from build123d import *

# Parameters (mm, degrees)
SKETCH_1_R      = 4.025
EXTRUDE_1_DEPTH = 1.5
FILLET_1_R      = 13
FILLET_2_R      = 6
FILLET_3_R      = 1
FILLET_7_R      = 3


with BuildPart() as part:
    # 草图1 → 凸台-拉伸1 (new, symmetric)
    with BuildSketch(Plane.XY):
        with BuildLine():
            Line((38, 14.000000007), (250, 10.55184781))
            ThreePointArc((250, 10.55184781), (369.998701007, 8.688014918), (490.000004009, 7))
            ThreePointArc((490.000004009, 7), (564.99833736, 6.250002778), (640.000004009, 6))
            Line((640.000004009, 6), (750.000004009, 6))
            ThreePointArc((750.000004009, 6), (767.416160301, 6.375174017), (784.800004009, 7.5))
            ThreePointArc((784.800004009, 7.5), (788.089261415, 6.498216371), (789.772556789, 3.5))
            ThreePointArc((789.772556789, 3.5), (790.000004009, 0), (789.772556789, -3.5))
            ThreePointArc((789.772556789, -3.5), (788.089261415, -6.498216371), (784.800004009, -7.5))
            ThreePointArc((784.800004009, -7.5), (767.416160301, -6.375174017), (750.000004009, -6))
            Line((750.000004009, -6), (640.000004009, -6))
            ThreePointArc((640.000004009, -6), (564.99833736, -6.250002778), (490.000004009, -7))
            ThreePointArc((490.000004009, -7), (369.998701007, -8.688014918), (250, -10.55184781))
            Line((250, -10.55184781), (38, -14.000000007))
            Line((38, -14.000000007), (30.845299463, -26.392304848))
            Line((30.845299463, -26.392304848), (26, -18))
            Line((26, -18), (14.154700538, -38.516660498))
            Line((14.154700538, -38.516660498), (24.248711306, -56))
            Line((24.248711306, -56), (29.856406461, -56))
            Line((29.856406461, -56), (35.052558882, -65))
            Line((35.052558882, -65), (19.052558883, -65))
            Line((19.052558883, -65), (3.649147039, -38.320508076))
            Line((3.649147039, -38.320508076), (-0.207259422, -45))
            Line((-0.207259422, -45), (2.596588156, -49.856406461))
            Line((2.596588156, -49.856406461), (-2.599564267, -58.856406461))
            Line((-2.599564267, -58.856406461), (-10.599564267, -45))
            Line((-10.599564267, -45), (-1.547005384, -29.320508076))
            Line((-1.547005384, -29.320508076), (-11.547005384, -12))
            ThreePointArc((-11.547005384, -12), (-19.547005384, -11), (-27.547005384, -12))
            ThreePointArc((-27.547005384, -12), (-90.773502692, -16), (-154, -12))
            ThreePointArc((-154, -12), (-162, -11), (-170, -12))
            Line((-170, -12), (-175.773502692, -22))
            Line((-175.773502692, -22), (-187.226497308, -22))
            Line((-187.226497308, -22), (-193, -12))
            Line((-193, -12), (-203.07179677, -12))
            Line((-203.07179677, -12), (-210, 0))
            Line((-210, 0), (-203.071796768, 12))
            Line((-203.071796768, 12), (-193, 12))
            Line((-193, 12), (-187.226497308, 22))
            Line((-187.226497308, 22), (-175.773502689, 22))
            Line((-175.773502689, 22), (-170, 12))
            ThreePointArc((-170, 12), (-162, 11), (-154, 12))
            ThreePointArc((-154, 12), (-90.773502692, 16), (-27.547005384, 12))
            ThreePointArc((-27.547005384, 12), (-19.547005384, 11), (-11.547005384, 12))
            Line((-11.547005384, 12), (-1.547005384, 29.320508076))
            Line((-1.547005384, 29.320508076), (-10.599564267, 45))
            Line((-10.599564267, 45), (-2.599564267, 58.856406461))
            Line((-2.599564267, 58.856406461), (2.596588156, 49.856406461))
            Line((2.596588156, 49.856406461), (-0.207259422, 45))
            Line((-0.207259422, 45), (3.649147039, 38.320508076))
            Line((3.649147039, 38.320508076), (19.052558883, 65))
            Line((19.052558883, 65), (35.052558883, 65))
            Line((35.052558883, 65), (29.856406461, 56))
            Line((29.856406461, 56), (24.248711306, 56))
            Line((24.248711306, 56), (14.154700538, 38.516660498))
            Line((14.154700538, 38.516660498), (26, 18))
            Line((26, 18), (30.845299464, 26.392304849))
            Line((30.845299464, 26.392304849), (38, 14.000000007))
        make_face()
        with Locations((-120.773502692, 0)):
            Circle(SKETCH_1_R, mode=Mode.SUBTRACT)
        with Locations((-60.773502692, 0)):
            Circle(SKETCH_1_R, mode=Mode.SUBTRACT)
        with Locations((-180.773502692, 0)):
            Circle(SKETCH_1_R, mode=Mode.SUBTRACT)
        with Locations((5.226497308, 0)):
            Circle(SKETCH_1_R, mode=Mode.SUBTRACT)
        Polygon((-206, 0), (-203.690598923, 4), (-199.07179677, 4), (-196.762395693, 0), (-199.07179677, -4), (-203.690598923, -4), align=None, mode=Mode.SUBTRACT)
    extrude(amount=EXTRUDE_1_DEPTH, both=True)

    # 圆角1
    fillet_1_edges = [part.edges().sort_by_distance(p)[0] for p in [
        (-1.547005384, -29.320508076, 0),
        (-11.547005384, -12, 0),
        (-170, -12, 0),
        (-170, 12, 0),
        (-11.547005384, 12, 0),
        (-1.547005384, 29.320508076, 0),
    ]]
    fillet(fillet_1_edges, radius=FILLET_1_R)

    # 圆角2
    fillet_2_edges = [part.edges().sort_by_distance(p)[0] for p in [
        (14.154700538, -38.516660498, 0),
        (19.052558883, -65, 0),
        (-10.599564267, -45, 0),
        (-10.599564267, 45, 0),
        (19.052558883, 65, 0),
        (14.154700538, 38.516660498, 0),
    ]]
    fillet(fillet_2_edges, radius=FILLET_2_R)

    # 圆角3
    fillet_3_edges = [part.edges().sort_by_distance(p)[0] for p in [
        (-196.762395693, 0, 0),
        (-199.07179677, 4, 0),
        (-203.690598923, 4, 0),
        (-206, 0, 0),
        (-203.690598923, -4, 0),
        (-199.07179677, -4, 0),
        (24.248711306, -56, 0),
        (29.856406461, -56, 0),
        (35.052558882, -65, 0),
        (3.649147039, -38.320508076, 0),
        (-0.207259422, -45, 0),
        (2.596588156, -49.856406461, 0),
        (-2.599564267, -58.856406461, 0),
        (-2.599564267, 58.856406461, 0),
        (2.596588156, 49.856406461, 0),
        (-0.207259422, 45, 0),
        (3.649147039, 38.320508076, 0),
        (35.052558883, 65, 0),
        (29.856406461, 56, 0),
        (24.248711306, 56, 0),
        (26, 18, 0),
        (30.845299464, 26.392304849, 0),
        (30.845299463, -26.392304848, 0),
        (26, -18, 0),
    ]]
    fillet(fillet_3_edges, radius=FILLET_3_R)

    # 圆角5
    # a fillet whose section is not a circle: 12, 9 mm, written as the material it adds along each edge
    with BuildSketch(Plane(origin=(38, -14.000000007, 1.5), x_dir=(0.9998677532589965, 0.016262717878828103, 0), z_dir=(0, 0, -1))) as fillet_5_piece_1:
        with BuildLine():
            Bezier((8.596427908, 0), (0, 0), (-1.696926281, 2.831786358), weights=[1, 1, 1])
            Line((-1.696926281, 2.831786358), (0, 0))
            Line((0, 0), (8.596427908, 0))
        make_face()
    extrude(amount=3)

    # 圆角6
    # a fillet whose section is not a circle: 12, 9 mm, written as the material it adds along each edge
    with BuildSketch(Plane(origin=(38, 14.000000007, 1.5), x_dir=(-0.5000000000000278, 0.8660254037844227, 0), z_dir=(0, 0, -1))) as fillet_6_piece_1:
        with BuildLine():
            Bezier((3.301298651, 0), (0, 0), (-4.418716991, 7.373839769), weights=[1, 1, 1])
            Line((-4.418716991, 7.373839769), (0, 0))
            Line((0, 0), (3.301298651, 0))
        make_face()
    extrude(amount=3)

    # 圆角7
    fillet_7_edges = [part.edges().sort_by_distance(p)[0] for p in [
        (-175.773502692, -22, 0),
        (-187.226497308, -22, 0),
        (-193, -12, 0),
        (-203.07179677, -12, 0),
        (-210, 0, 0),
        (-203.071796768, 12, 0),
        (-193, 12, 0),
        (-187.226497308, 22, 0),
        (-175.773502689, 22, 0),
    ]]
    fillet(fillet_7_edges, radius=FILLET_7_R)


solid = part.part
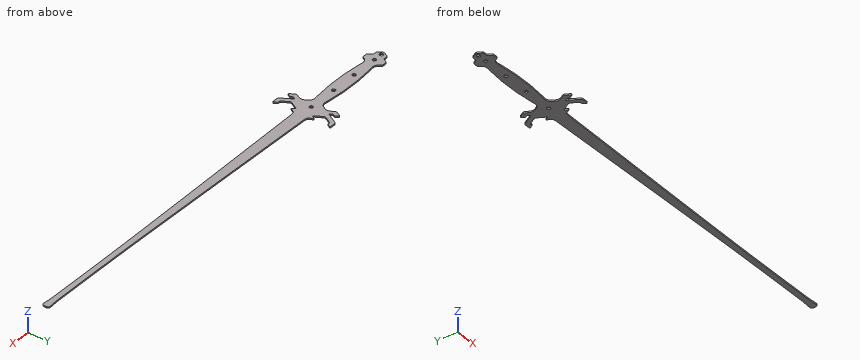
The listing builds one solid part. Answer for the finished solid, in the listing's coordinates (mm). Round coordinates to 2 decimals unless told otherwise and drop trailing zeros. Write each loop counter-clockwise with the first axis right and the second up, starting at its lowest first coordinate (ties: lowest second). Pieces come first, ordered by that corner, then holes. Notation, with made-up numbers: (8, 35.5) - (53, 35.5) arc R28 cw to (53, 58.5) - close; hole circle Ø6 at (-5.75, 47). An arc over 180 degrees is marked (long way). Use a Markdown table: item, result. Add a question column.
1. The part is cut by section B-B (x = 176.5). Write down the section's boundary in (y, z), and give its area (3 significant figures).
2. Flat-ended cylindrical pins translate along their axes: P1, Ø1.5, axis at x = -197.5, z = 0, coming from the +Y side; P2, Ø0.9, axis at x = -182, z = -0.5, coming from the +Y side; P3, Ø0.9, axis at x = 693.5, z = 0.5, coming from the +Y side. Find the tip coordinate at first contact, or state that the pin passes through.
3. Consider line 1 (X direction, y = -44, z = 1.3); line 2 (Y direction, x = 496.5, z = 0.75); line 3 (X direction, y = -30, z = -0.1). Determine where each line is inside the solid, lowest interval first.
4. The part is cut by section A-A (z = -0.4). Give the number of separate pieces and of enclosed holes in the cut face, and give its area (3 significant figures).
Reported:
| question | item | result |
|---|---|---|
| 1 | outline | (-11.75, -1.5) - (11.75, -1.5) - (11.75, 1.5) - (-11.75, 1.5) - close |
| 1 | area | 70.5 mm^2 |
| 2 | P1 | y = 12 |
| 2 | P2 | y = 22 |
| 2 | P3 | y = 6 |
| 3 | line 1 | -9.59 to 0.37, 6.93 to 17.32 |
| 3 | line 2 | -6.92 to 6.92 |
| 3 | line 3 | -3.58 to 19.07 |
| 4 | separate pieces | 1 |
| 4 | enclosed holes | 5 |
| 4 | area | 22,400 mm^2 |
